```python
from build123d import *

# Parameters (mm, degrees)
F1_DEPTH = 870
F2_T     = -25


with BuildPart() as f1:
    # F0 (on Front) → F1 (new body)
    with BuildSketch(Plane.XZ):
        Polygon((315.272604, -122.337317), (263.946945, 122.337317), (126.402124, 182.182302), (-22.584686, 199.587198), (-149.872822, 120.228958), (-202.089188, -20.389146), (-131.931266, -260.343029), (11.636889, -303.796281), (155.66179, -345.710812), (284.671261, -269.18267), align=None)
    extrude(amount=F1_DEPTH)

    # F2
    f2_openings = [f1.faces().sort_by_distance(p)[0] for p in [
        (64.144057, -870, -68.345296),
    ]]
    offset(amount=F2_T, openings=f2_openings)


solid = f1.part
```
Geometry: final body of the model. Coordinates: model frame, mm. A direction names the side the tool comes from. Give positions to 0.01 mm unless a question says otherwise; leave off trailing zeros. Order: outer loops, then holes, each group sorted by start corner. A loop starts at its lowest first (then second) coordinate and runs counter-clockwise, first axis right, second up. Notation, with made-up numbers: M 22,64.25 L 56,64.25 A16 ccw 56,79.25 Z; hole C -20,30 d11. An arc over 180 degrees is marked long. Answer as CSV lines item,"result". Start each with the question number.
1) Line query: line 1 (Y direction, x = 230, z = 26); line 2 (X direction, y = -391, z = -32.5); line 3 (Z direction, x = 240, y = -728). Output: solid intervals per line, ascending. Write a range as from..to.
2) Cut plane C-C (z = -50). Output: boundary loops of the cut face in (x, y), then the cut area to 3 significant figures.
3) Cut plane B-B (x = -81.5). Output: boundary loops of the cut face in (y, z), then the cut area to 3 significant figures.
4) Cut plane A-A (y = -513). Output: boundary loops of the cut face in (x, z).
5) Set-up query: faces 1 (the flat face through (-72.309, -441.585, 139.126)), 2 (the flat face through (196.14, -428.91, 151.84)). Return all of +Z, -Z, +X, -X, +Y, -Y with unobstructed straight access to the full face (end or side cutting, diameter ignored); none if empty.
6) First-contact query: P1, Ø8, axis at x = 99, y = -449, coming from the -Z side; P2, Ø8, axis at x = -118, y = -167, coming from the +Z side; P3, Ø10, axis at y = -184.5, z = 59.5, coming from the -X side; P4, Ø5, axis at x = 157.5, z = 103.5, coming from the +Y side. Flat tips, straight axial feed; report the tip coordinate or a pass-through.
7) Mould query, pull axis X, two halves, no side actions, for faces 3 (the flat face through (-61.152, -428.91, -281.765)), 4 (the flat face through (52.952, -428.91, 190.763)), 5 (the flat face through (-144.2, -441.6, -129.3)). Classes: +X half, -X half, draft (parallel to the pull), parting line (faces both ways), or undercut.
Findings below:
1,line 1,"y = -25..0"
1,line 2,"x = -198.55..-172.5, 270.88..296.43"
1,line 3,"z = -295.68..-266.61, 105.49..132.76"
2,outline,"M -193.43,-870 L -167.38,-870 L -167.38,-25 L 274.55,-25 L 274.55,-870 L 300.1,-870 L 300.1,0 L -193.43,0 Z"
2,area,"55,900 mm²"
3,outline,"M -870,-275.61 L 0,-275.61 L 0,162.86 L -870,162.86 L -870,133.4 L -25,133.4 L -25,-249.49 L -870,-249.49 Z"
3,area,"57,900 mm²"
4,outline,"M -202.09,-20.39 L -131.93,-260.34 L 11.64,-303.8 L 155.66,-345.71 L 284.67,-269.18 L 315.27,-122.34 L 263.95,122.34 L 126.4,182.18 L -22.58,199.59 L -149.87,120.23 Z; hole M -175.77,-21.33 L -111.73,-240.34 L 18.75,-279.83 L 152.23,-318.68 L 262.44,-253.3 L 289.73,-122.35 L 242.13,104.57 L 119.82,157.78 L -16.79,173.74 L -129.41,103.53 Z"
5,face 1,"-Y"
5,face 2,"+Z, +X, +Y, -Y"
6,P1,"stops at z = -330.39"
6,P2,"stops at z = 142.59"
6,P3,"stops at x = -174.28"
6,P4,"stops at y = 0"
7,face 3,"-X half"
7,face 4,"+X half"
7,face 5,"undercut"
